Verification items for this drawing (mm, ordinates from the low corner). A direction names the side the tool comes from. Round coordinates to 2 decimals unless told otherwise and drop trailing zeros. Write each loop counter-clockwise with the first axis right and the second up, starting at its lowest first coordinate (ties: lowest second). Pieces come first, ordered by that corner, then holes. Notation, with made-up numbers: (1, 37.5) -> (53, 37.5) arc R27 cw to (53, 66.5) -> close; hole circle Ø9 at (16.25, 32). An arc over 180 degrees is marked (long way). One line per question, with ' | ' between items.
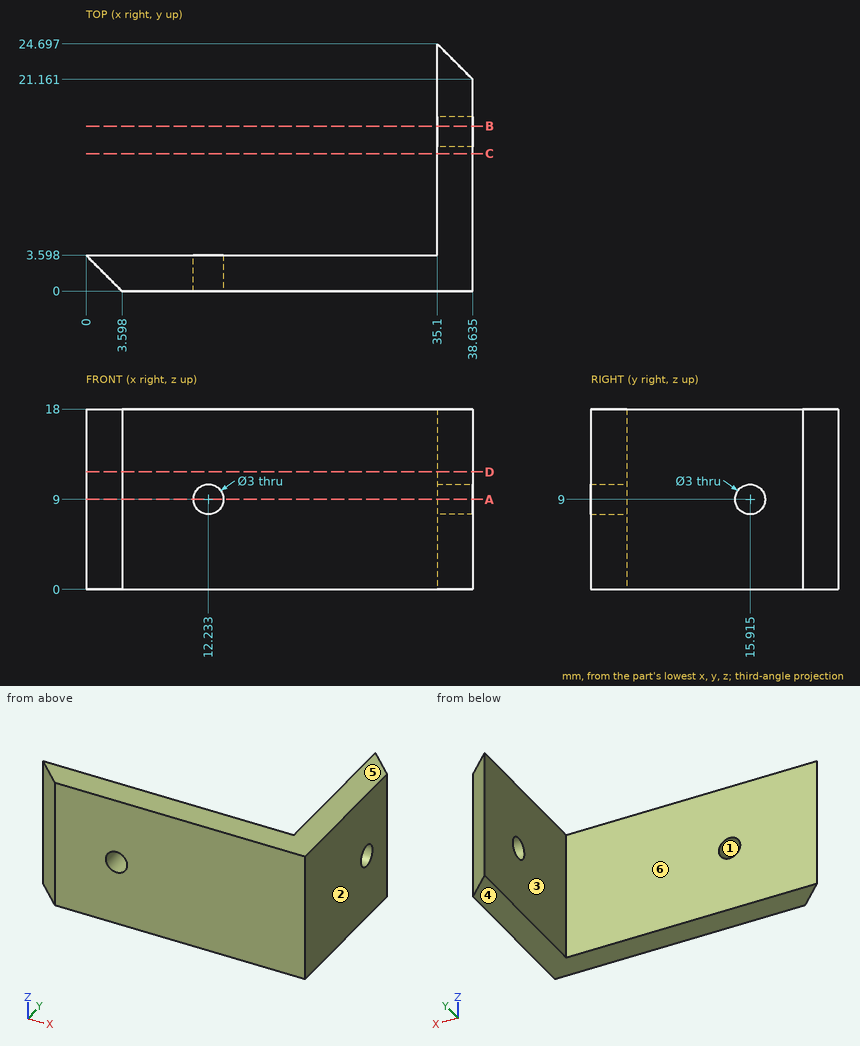
(1) Sectioned sample at D-D on z = 11.75. Record the cut outline in (x, y) (1 decimal).
Resolved:
outline: (0, 3.6) -> (3.6, 0) -> (38.6, 0) -> (38.6, 21.2) -> (35.1, 24.7) -> (35.1, 3.6) -> close
(2) Sectioned sample at C-C on y = 13.75. Record the cut outline in (x, z) (1 decimal).
Resolved:
outline: (35.1, 0) -> (38.6, 0) -> (38.6, 18) -> (35.1, 18) -> close
(3) Draft check along X on the marked faces 1, 2, 3 and 4. Enter one of: +X half, -X half, draft (parallel to the pull), parting line (faces both ways), or undercut.
Resolved:
face 1: undercut | face 2: +X half | face 3: -X half | face 4: draft
(4) Sectioned sample at A-A on z = 9. Record the cut outline in (x, y) (1 decimal).
Resolved:
outline: (0, 3.6) -> (3.6, 0) -> (10.7, 0) -> (10.7, 3.6) -> close; (13.7, 0) -> (38.6, 0) -> (38.6, 14.4) -> (35.1, 14.4) -> (35.1, 3.6) -> (13.7, 3.6) -> close; (35.1, 17.4) -> (38.6, 17.4) -> (38.6, 21.2) -> (35.1, 24.7) -> close
(5) Sectioned sample at B-B on y = 16.5. Record the cut outline in (x, z) (1 decimal).
Resolved:
outline: (35.1, 0) -> (38.6, 0) -> (38.6, 7.6) -> (35.1, 7.6) -> close; (35.1, 10.4) -> (38.6, 10.4) -> (38.6, 18) -> (35.1, 18) -> close
(6) Material ranges on line 1 (Y direction, x = 21.5, z = 7.75); line 2 (Y direction, x = 37.6, z = 9) (1 decimal); line 3 (X direction, y = 7, z = 12) (1 decimal), recorded low to high.
Resolved:
line 1: y = 0 to 3.6 | line 2: y = 0 to 14.4, 17.4 to 22.2 | line 3: x = 35.1 to 38.6
(7) Access from +Z, -Z, +X, -X, +Y, -Y to the whole of each face (thin tool, end or side, straight path). Record for the marked faces 5 and 6.
Resolved:
face 5: +Z, +X, -X, +Y, -Y | face 6: +Z, -Z, -X, +Y
(8) Go/stop test with flat-tipped pins: pin 1 (1 mm diameter, centred on x = 16, z = 10, fed in from +Y); pin 2 (12 mm diameter, centred on x = 7.5, y = 14.5, fed in from -Z); pin 3 (9 mm diameter, centred on y = 16, z = 11.5, fed in from -X). Record where each tip stops, or that it passes through.
Resolved:
pin 1: stops at y = 3.6 | pin 2: passes through | pin 3: stops at x = 35.1
